Build history of the part. All positions in model axes, mm. A direction names the side the tool comes from. Coordinates: 2 decimals unless noted, no trailing zeros. Order: outer loops, then holes, each group sorted by start corner. A loop starts at its lowest first (then second) coordinate and runs counter-clockwise, first axis right, second up. Notation, with made-up numbers: (-15, -1.5) - (18, -1.5) arc R11 ccw to (18, 16.5) - close; hole circle Ø3 at (29, 58.25). An arc over 180 degrees is marked (long way). Answer as CSV lines item,"result". Start each with the question number.
from build123d import *

# Parameters (mm, degrees)
SKETCH_R  = 3.35
PAD_DEPTH = 93


with BuildPart() as part:
    # Sketch → Pad (new body)
    with BuildSketch(Plane.XY):
        with BuildLine():
            Line((20, 1), (-2.5, 1))
            Line((-2.5, 1), (-2.5, 0))
            Line((0, 0), (-2.5, 0))
            Line((0, -10), (0, 0))
            ThreePointArc((0, -10), (5, -15), (10, -10))
            Line((10, -10), (10, -1))
            Line((10, -1), (19, -1))
            Line((19, -1), (19, -5))
            Line((19, -5), (20, -5))
            Line((20, -5), (20, 1))
        make_face()
        with Locations((5, -10)):
            Circle(SKETCH_R, mode=Mode.SUBTRACT)
    extrude(amount=PAD_DEPTH)


solid = part.part
(1) Band-saw the part on A-A on x = 5. List the corners of the cut face in (y, z).
(2) Band-saw the part on D-D on x = -1. List the corners of the cut face in (y, z), plus the area to 3 significant figures.
(3) Drop flat-ended pins along their axis: pin 1 Ø0.8 at (x, z) = (19.5, 53.5) entering from -Y; pin 2 Ø5 at (y, z) = (-11.5, 71.5) entering from +X; pin 3 Ø4 at (x, z) = (14.5, 66.5) entering from -Y; pin 4 Ø1 at (x, y) = (11, -9) entering from +Z. Give the stop position or say it passes through.
(4) Which spindle directions (+Z, -Z, +X, -X, +Y, -Y) get a long thin tool onto all of the face, cutting with end or side? Do faces 5 (the flat face through (10, -6, 46)), 6 (the flat face through (-1, 0, 46)), 7 (the flat face through (9, 1, 46)). Say none if no direction does.
(5) Pull direction X, two halves, no side cores. Call faces 1 (the cylindrical face through (6.55, -12.97, 45.85)), 2 (the flat face through (0, -5, 46)), 3 (the flat face through (6, -5, 93)), 4 (the flat face through (20, -2, 46)): +X half, -X half, draft (parallel to the pull), parting line (faces both ways), or undercut.
(6) Band-saw the part on C-C on z = 34. List the corners of the cut face in (x, y), plus the area to 3 significant figures.
(7) Probe L1, parallel to X at y = -2, z = 16.5; L2, parallel to Y at x = 5, z = 56; L3, parallel to Y at x = 11.5, z = 81. List the from-to ranges inside material, lowest first. Write a range as [from, to].
(8) Band-saw the part on B-B on y = -4. List the corners of the cut face in (x, z), plus the area to 3 significant figures.
Filled in:
1,outline,"(-15, 0) - (-13.35, 0) - (-13.35, 93) - (-15, 93) - close; (-6.65, 0) - (1, 0) - (1, 93) - (-6.65, 93) - close"
2,outline,"(0, 0) - (1, 0) - (1, 93) - (0, 93) - close"
2,area,"93.0 mm^2"
3,pin 1,"stops at y = -5"
3,pin 2,"stops at x = 10"
3,pin 3,"stops at y = -1"
3,pin 4,"passes through"
4,face 5,"+Z, -Z, -Y"
4,face 6,"+Z, -Z, -X, -Y"
4,face 7,"+Z, -Z, +X, -X, +Y"
5,face 1,"undercut"
5,face 2,"-X half"
5,face 3,"draft"
5,face 4,"+X half"
6,outline,"(-2.5, 0) - (0, 0) - (0, -10) arc R5 ccw to (10, -10) - (10, -1) - (19, -1) - (19, -5) - (20, -5) - (20, 1) - (-2.5, 1) - close; hole circle Ø6.7 at (5, -10)"
6,area,"141 mm^2"
7,L1,"x = [0, 10], [19, 20]"
7,L2,"y = [-15, -13.35], [-6.65, 1]"
7,L3,"y = [-1, 1]"
8,outline,"(0, 0) - (10, 0) - (10, 93) - (0, 93) - close; (19, 0) - (20, 0) - (20, 93) - (19, 93) - close"
8,area,"1,020 mm^2"
